Build history of the part. All positions in model axes, mm. Coordinates: 2 decimals unless noted, no trailing zeros. Write each loop counter-clockwise with the first axis right and the second up, starting at its lowest first coordinate (ties: lowest second). Pieces come first, ordered by that corner, then holes.
from build123d import *

# Parameters (mm, degrees)
CROQUIS2_W              = 30
CROQUIS2_H              = 20
SALIENTE_EXTRUIR2_DEPTH = 25
SALIENTE_EXTRUIR3_DEPTH = 30
REDONDEO1_R             = 5
CROQUIS8_R              = 1.5
CORTAR_EXTRUIR5_DEPTH   = 26
CROQUIS9_R              = 1.5
CORTAR_EXTRUIR6_DEPTH   = 32.819805153


with BuildPart() as part:
    # Croquis2 → Saliente-Extruir2 (new body)
    with BuildSketch(Plane(origin=(0, 0, 0), x_dir=(0, 0, -1), z_dir=(1, 0, 0))):
        with Locations((-15, -10)):
            Rectangle(CROQUIS2_W, CROQUIS2_H)
    extrude(amount=SALIENTE_EXTRUIR2_DEPTH)

    # Croquis3 → Saliente-Extruir3 (add, through all)
    with BuildSketch(Plane(origin=(0, 0, 0), x_dir=(-1, 0, 0), z_dir=(0, 0, -1))):
        Polygon((0, 0), (0, 25), (-25, 0), align=None)
    extrude(amount=-SALIENTE_EXTRUIR3_DEPTH)

    # Redondeo1
    redondeo1_edges = [part.edges().sort_by_distance(p)[0] for p in [
        (0, 25, 15),
    ]]
    fillet(redondeo1_edges, radius=REDONDEO1_R)

    # Croquis8 → Cortar-Extruir5 (cut, through all)
    with BuildSketch(Plane.ZY):
        with Locations((20, -10)):
            Circle(CROQUIS8_R)
        with Locations((5, -10)):
            Circle(CROQUIS8_R)
    extrude(amount=-CORTAR_EXTRUIR5_DEPTH, mode=Mode.SUBTRACT)

    # Croquis9 → Cortar-Extruir6 (cut, through all)
    with BuildSketch(Plane(origin=(12.5, 12.5, 0), x_dir=(0, 0, -1), z_dir=(0.707106781, 0.707106781, 0))):
        with Locations((-16.056627864, -2.050053866)):
            Circle(CROQUIS9_R)
        with Locations((-5.000664805, -2.050053866)):
            Circle(CROQUIS9_R)
    extrude(amount=-CORTAR_EXTRUIR6_DEPTH, mode=Mode.SUBTRACT)


solid = part.part
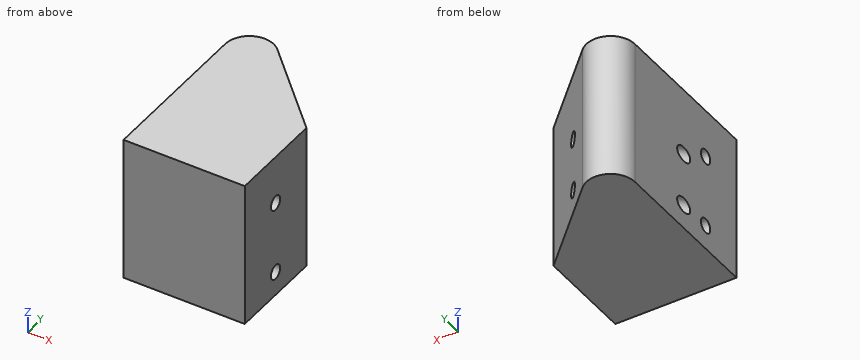
(1) Flat gauge pins, fed straight in: P1, Ø3.5, axis at y = -10, z = 20, coming from the -X side; P2, Ø3, axis at x = 10, z = 6, coming from the +Y side. Where does each tip first touch, or does it go through?
(2) Slice it at A-A, the plane y = -10. List the corners of the cut face in (x, z), and give its area (3 significant figures).
(3) Slice it at D-D, the plane z = 5. List the corners of the cut face in (x, y).
(4) Slice it at C-C, the plane x = 20. List the corners of the cut face in (y, z).
(5) Slice it at B-B, the plane z = 15.5. List the corners of the cut face in (x, y), and give its area (3 significant figures).
(6) Probe L1, parallel to Z at x = 5, y = -11; L2, parallel to Z at x = 23.25, y = -9.5; L3, parallel to Y at x = 10, z = 19.5. List the from-to ranges inside material, lowest first.
Results:
1. P1: stops at x = 0
1. P2: stops at y = 16.5
2. outline: (0, 0) - (25, 0) - (25, 3.5) - (0, 3.5) - close; (0, 6.5) - (25, 6.5) - (25, 18.5) - (0, 18.5) - close; (0, 21.5) - (25, 21.5) - (25, 30) - (0, 30) - close
2. area: 600 mm2
3. outline: (0, -20) - (25, -20) - (25, -11.5) - (0, -11.5) - close; (0, -8.5) - (25, -8.5) - (25, 0) - (15.01, 9.99) - (0, -5.02) - close; (0, -0.78) - (12.89, 12.11) - (8.54, 16.46) arc R5 ccw to (0, 12.93) - close
4. outline: (-20, 0) - (5, 0) - (5, 30) - (-20, 30) - close; hole circle Ø3 at (-10, 5); hole circle Ø3 at (-10, 20)
5. outline: (0, -20) - (25, -20) - (25, 0) - (14.93, 10.07) - (0, -4.87) - close; (0, -0.93) - (12.96, 12.04) - (8.54, 16.46) arc R5 ccw to (0, 12.93) - close
5. area: 727 mm2
6. L1: z = 0 to 3.88, 6.12 to 18.88, 21.12 to 30
6. L2: z = 0 to 3.59, 6.41 to 18.59, 21.41 to 30
6. L3: y = -20 to -11.41, -8.59 to 15
